```python
from build123d import *

# Parameters (mm, degrees)
F1_DEPTH = 18
F3_DEPTH = 25
F5_DEPTH = 18
F6_W     = 16
F6_H     = 4
F7_DEPTH = 600
F9_D     = 6
F9_DEPTH = 8
F9_TIP   = 1.8025818571


with BuildPart() as f1:
    # F0 (on Front) → F1 (new body)
    with BuildSketch(Plane.XZ):
        with BuildLine():
            Line((112.5127500061, 30.0339285255), (112.5127500061, 43.0339285255))
            Line((112.5127500061, 43.0339285255), (3.8390576642, 43.0339285255))
            Line((3.8390576642, 43.0339285255), (0.8390576642, 40.0339285255))
            Line((0.8390576642, 40.0339285255), (0.8390576642, 25.0339285255))
            ThreePointArc((0.8390576642, 25.0339285255), (-0.6254084298, 21.4983946196), (-4.1609423358, 20.0339285255))
            Line((-4.1609423358, 20.0339285255), (-34.1609423358, 20.0339285255))
            ThreePointArc((-34.1609423358, 20.0339285255), (-36.9560273076, 20.8881475376), (-38.7960663902, 23.1589285255))
            Line((-38.7960663902, 23.1589285255), (-41.5771408229, 25.0339285255))
            Line((-41.5771408229, 25.0339285255), (-58.7447438487, 25.0339285255))
            Line((-58.7447438487, 25.0339285255), (-61.5258182813, 23.1589285255))
            ThreePointArc((-61.5258182813, 23.1589285255), (-63.3658573639, 20.8881475376), (-66.1609423358, 20.0339285255))
            Line((-66.1609423358, 20.0339285255), (-96.1609423358, 20.0339285255))
            ThreePointArc((-96.1609423358, 20.0339285255), (-99.6964762417, 21.4983946196), (-101.1609423358, 25.0339285255))
            Line((-101.1609423358, 25.0339285255), (-101.1609423358, 40.0339285255))
            Line((-101.1609423358, 40.0339285255), (-104.1609423358, 43.0339285255))
            Line((-104.1609423358, 43.0339285255), (-228.6609423358, 43.0339285255))
            Line((-228.6609423358, 43.0339285255), (-228.6609423358, 30.0339285255))
            ThreePointArc((-228.6609423358, 30.0339285255), (-230.1254084298, 26.4983946196), (-233.6609423358, 25.0339285255))
            Line((-233.6609423358, 25.0339285255), (-238.6609423358, 25.0339285255))
            ThreePointArc((-238.6609423358, 25.0339285255), (-242.1964762417, 26.4983946196), (-243.6609423358, 30.0339285255))
            Line((-243.6609423358, 30.0339285255), (-243.6609423358, 43.0339285255))
            Line((-243.6609423358, 43.0339285255), (-298.1612311549, 43.0339285255))
            Line((-298.1612311549, 43.0339285255), (-298.1612311549, 3.0339285255))
            Line((-298.1612311549, 3.0339285255), (94.8881047238, 3.0339285255))
            Line((94.8881047238, 3.0339285255), (94.8881047238, 7.0339285255))
            Line((94.8881047238, 7.0339285255), (152.5947688451, 7.0339285255))
            Line((152.5947688451, 7.0339285255), (152.5947688451, 20.0339285255))
            Line((152.5947688451, 20.0339285255), (89.8390576642, 20.0339285255))
            ThreePointArc((89.8390576642, 20.0339285255), (84.8390576642, 25.0339285255), (89.8390576642, 30.0339285255))
            Line((89.8390576642, 30.0339285255), (112.5127500061, 30.0339285255))
        make_face()
        with BuildLine():
            ThreePointArc((-282.1609423358, 20.0339285255), (-287.1609423358, 25.0339285255), (-282.1609423358, 30.0339285255))
            Line((-282.1609423358, 30.0339285255), (-252.1609423358, 30.0339285255))
            ThreePointArc((-252.1609423358, 30.0339285255), (-247.1609423358, 25.0339285255), (-252.1609423358, 20.0339285255))
            Line((-252.1609423358, 20.0339285255), (-282.1609423358, 20.0339285255))
        make_face(mode=Mode.SUBTRACT)
        with BuildLine():
            ThreePointArc((-220.1609423358, 20.0339285255), (-225.1609423358, 25.0339285255), (-220.1609423358, 30.0339285255))
            Line((-220.1609423358, 30.0339285255), (-190.1609423358, 30.0339285255))
            ThreePointArc((-190.1609423358, 30.0339285255), (-185.1609423358, 25.0339285255), (-190.1609423358, 20.0339285255))
            Line((-190.1609423358, 20.0339285255), (-220.1609423358, 20.0339285255))
        make_face(mode=Mode.SUBTRACT)
        with BuildLine():
            ThreePointArc((-158.1609423358, 20.0339285255), (-163.1609423358, 25.0339285255), (-158.1609423358, 30.0339285255))
            Line((-158.1609423358, 30.0339285255), (-128.1609423358, 30.0339285255))
            ThreePointArc((-128.1609423358, 30.0339285255), (-123.1609423358, 25.0339285255), (-128.1609423358, 20.0339285255))
            Line((-128.1609423358, 20.0339285255), (-158.1609423358, 20.0339285255))
        make_face(mode=Mode.SUBTRACT)
        with BuildLine():
            ThreePointArc((27.8390576642, 20.0339285255), (22.8390576642, 25.0339285255), (27.8390576642, 30.0339285255))
            Line((27.8390576642, 30.0339285255), (57.8390576642, 30.0339285255))
            ThreePointArc((57.8390576642, 30.0339285255), (62.8390576642, 25.0339285255), (57.8390576642, 20.0339285255))
            Line((57.8390576642, 20.0339285255), (27.8390576642, 20.0339285255))
        make_face(mode=Mode.SUBTRACT)
    extrude(amount=F1_DEPTH)

    # F2 (on face) → F3 (cut)
    with BuildSketch(Plane.XY.offset(20.0339285255)):
        Polygon((152.5947688451, -18), (152.5947688451, 0), (126.8877688451, 0), align=None)
    extrude(amount=-F3_DEPTH, mode=Mode.SUBTRACT)

    # F4 (on face) → F5 (cut)
    with BuildSketch(Plane.XY.offset(43.0339285255)):
        Polygon((112.5127500061, -18), (112.5127500061, 0), (102.4437500061, 0), align=None)
    extrude(amount=-F5_DEPTH, mode=Mode.SUBTRACT)

    # F6 (on face) → F7 (cut)
    with BuildSketch(Plane.YZ.offset(94.8881047238)):
        with Locations((-8, 5.0339285255)):
            Rectangle(F6_W, F6_H)
    extrude(amount=-F7_DEPTH, mode=Mode.SUBTRACT)

    # F9
    with Locations(Plane(origin=(0, 0, 7.0339285255), x_dir=(1, 0, 0), z_dir=(0, 0, -1))):
        with Locations((-186.1612311549, 11), (-6.1612311549, 11)):
            Hole(F9_D / 2, depth=F9_DEPTH)
            with Locations((0, 0, -(F9_DEPTH + F9_TIP / 2))):  # 118° drill point
                Cone(0, F9_D / 2, F9_TIP, mode=Mode.SUBTRACT)


solid = f1.part
```
Input: part model. Units: mm. Frame: model coordinates. A direction names the side the tool comes from. Round coordinates to 2 decimals unless told otherwise and drop trailing zeros. Order: outer loops, then holes, each group sorted by start corner. A loop starts at its lowest first (then second) coordinate and runs counter-clockwise, first axis right, second up. Notation, with made-up numbers: (72.5, 44) - (108.5, 44) arc R7 ccw to (108.5, 55) - close; hole circle Ø11 at (30, 3). An arc over 180 degrees is marked (long way). Answer in a Markdown table with one row per item.
Item 1: Mould query, pull axis Z, two halves, no side actions, for faces 6 (the flat face through (-243.661, -9, 36)), 7 (the cylindrical face through (-287.16, -8.87, 24.92)), 8 (the flat face through (-81, -9, 20.034)). Classes: released by +Z, released by -Z, zero draft, split by the parting line, or undercut.
Model answer:
| item | result |
|---|---|
| face 6 | zero draft |
| face 7 | undercut |
| face 8 | released by +Z |
Item 2: Section query C-C (y = -4). Give the number of separate pieces and of enclosed holes in the cut face, then the cut area to 3 significant figures.
Model answer:
| item | result |
|---|---|
| separate pieces | 1 |
| enclosed holes | 4 |
| area | 10,700 mm² |
Item 3: Section query A-A (z = 34). Return the cut outline in (x, y).
Model answer:
| item | result |
|---|---|
| outline | (-298.16, -18) - (-243.66, -18) - (-243.66, 0) - (-298.16, 0) - close; (-228.66, -18) - (-101.16, -18) - (-101.16, 0) - (-228.66, 0) - close; (0.84, -18) - (112.51, -18) - (102.44, 0) - (0.84, 0) - close |
Item 4: Section query B-B (x = -19). Return the cut outline in (y, z).
Model answer:
| item | result |
|---|---|
| outline | (-18, 3.03) - (-16, 3.03) - (-16, 7.03) - (0, 7.03) - (0, 20.03) - (-18, 20.03) - close |
Item 5: Line query: line 1 (Z direction, x = 50, y = -4.5); line 2 (X direction, y = -11, z = 10); line 3 (X direction, y = -4.5, z = 33.5). Output: solid intervals per line, ascending.
Model answer:
| item | result |
|---|---|
| line 1 | z = 7.03 to 20.03, 30.03 to 43.03 |
| line 2 | x = -298.16 to -189.16, -183.16 to -9.16, -3.16 to 142.6 |
| line 3 | x = -298.16 to -243.66, -228.66 to -101.16, 0.84 to 104.96 |
Item 6: Pin query (flat end, axial travel): pin 1 (5.5 mm diameter, centred on x = -266.5, y = -7.5, fed in from -Z); pin 2 (0.6 mm diameter, centred on y = -16.5, z = 4.5, fed in from +X); pin 3 (8.5 mm diameter, centred on x = -51.5, y = -5, fed in from +Z). Return the tip coordinate at first contact, or that it passes through.
Model answer:
| item | result |
|---|---|
| pin 1 | stops at z = 7.03 |
| pin 2 | stops at x = 94.89 |
| pin 3 | stops at z = 25.03 |
Item 7: Reachability of faces 1 (the flat face through (-298.161, -9, 23)), 2 (the flat face through (59, -9, 43.034)), 3 (the flat face through (-19, -9, 20.034)), 4 (the flat face through (98, -9, 30.034)), 5 (the cylindrical face through (-123.162, -8.874, 25.144)) from +Z, -Z, +X, -X, +Y, -Y: full face, straight path, thin tool, end or side. Return the list, or none.
Model answer:
| item | result |
|---|---|
| face 1 | +Z, -Z, -X, +Y, -Y |
| face 2 | +Z, +X, -X, +Y, -Y |
| face 3 | +Z, +Y, -Y |
| face 4 | +X, +Y, -Y |
| face 5 | +Y, -Y |
